```python
from build123d import *

# Parameters (mm, degrees)
BOSS_EXTRUDE1_DEPTH = 25
SHELL1_T            = -5
SKETCH3_W           = 5
SKETCH3_H           = 25
BOSS_EXTRUDE3_DEPTH = 5
CUT_EXTRUDE1_DEPTH  = 4.5


with BuildPart() as part:
    # Sketch1 → Boss-Extrude1 (new body)
    with BuildSketch(Plane(origin=(0, 0, 0), x_dir=(1, 0, 0), z_dir=(0, 1, 0))):
        Polygon((0, 42.5), (-36.806079661, 21.25), (-36.806079661, -21.25), (0, -42.5), (36.806079661, -21.25), (36.806079661, 21.25), align=None)
    extrude(amount=BOSS_EXTRUDE1_DEPTH)

    # Shell1
    shell1_openings = [part.faces().sort_by_distance(p)[0] for p in [
        (0, 25, 0),
        (-36.806079661, 12.5, 0),
    ]]
    offset(amount=SHELL1_T, openings=shell1_openings, kind=Kind.INTERSECTION)

    # Sketch3 → Boss-Extrude3 (add)
    with BuildSketch(Plane.XY.offset(-42.5)):
        with Locations((0, 12.5)):
            Rectangle(SKETCH3_W, SKETCH3_H)
    boss_extrude3 = extrude(amount=BOSS_EXTRUDE3_DEPTH)

    # Sketch4 → Cut-Extrude1 (cut)
    with BuildSketch(Plane(origin=(0, 0, -42.5), x_dir=(-1, 0, 0), z_dir=(0, 0, -1))):
        with BuildLine():
            ThreePointArc((0.573600046, 19.506352456), (1.318666007, 20.093843301), (1.6, 21))
            ThreePointArc((1.6, 21), (-0.906156699, 22.318666007), (-0.573600046, 19.506352456))
            ThreePointArc((-0.573600046, 19.506352456), (0, 19.71460041), (0.573600046, 19.506352456))
        make_face()
        with BuildLine():
            ThreePointArc((0.329089607, 2.434209455), (1.242284865, 2.991670533), (1.6, 4))
            ThreePointArc((1.6, 4), (-0.906156699, 5.318666007), (-0.573600046, 2.506352456))
            ThreePointArc((-0.573600046, 2.506352456), (-0.107313915, 2.657234104), (0.329089607, 2.434209455))
        make_face()
    cut_extrude1 = extrude(amount=-CUT_EXTRUDE1_DEPTH, mode=Mode.SUBTRACT)

    # Mirror1: Boss-Extrude3, Cut-Extrude1 across plane
    add(boss_extrude3.mirror(Plane.XY))
    add(cut_extrude1.mirror(Plane.XY), mode=Mode.SUBTRACT)


solid = part.part
```
Could you check a few things on this model? Use its own coordinates, in mm. A direction names the side the tool comes from. Give positions to 0.01 mm unless a question says otherwise; leave off trailing zeros. Write each loop counter-clockwise with the first axis right and the second up, starting at its lowest first coordinate (ties: lowest second). Pieces come first, ordered by that corner, then holes. Notation, with made-up numbers: (12.5, 65) - (34.5, 65) arc R18 cw to (34.5, 83) - close; hole circle Ø1 at (54.5, 80). An arc over 180 degrees is marked (long way). One line per item, written item: value. Start each with the question number.
Item 1: I'm going to push flat-ended pins straight in: pin 1 (0.7 mm diameter, centred on y = 7.5, z = -41.5, fed in from +X); pin 2 (0.9 mm diameter, centred on x = -0.5, y = 20.5, fed in from -Z); pin 3 (3.5 mm diameter, centred on x = 0, y = 21, fed in from -Z); pin 4 (1.5 mm diameter, centred on y = 3, z = 27, fed in from +X). Where does each tip first touch, or does it pass through?
Item 2: Imagine slicing it at D-D, the plane z = -33. List the corners of the cut face in (x, y) for me, and give its area (3 significant figures).
Item 3: Please list where these lines run through material, in increasing order: line 1 (Y direction, x = 0, z = -39); line 2 (X direction, y = 21, z = -41.45); line 3 (X direction, y = 16, z = -7.5). Write a range as from..to.
Item 4: Which directions (+Z, -Z, +X, -X, +Y, -Y) give clear straight access to the entire face, cutting with the end or side of a thin tool? Please do faces 4 (the face through (0, 21, 38)), 5 (the face through (-3, 5, -1)), 6 (the face through (0, 4, -38)).
Item 5: If we mould it in two halves opening along Y, with no side actions, what happens to faces 1 (the face through (22, 25, -25)), 2 (the face through (0, 4, 38)), 3 (the face through (-18.145, 14.86, -26.25))? For each: +Y half, -Y half, draft (parallel to the pull), parting line (faces both ways), or undercut.
Item 6: Imagine slicing it at A-A, the plane y = 10.5. List the corners of the cut face in (x, z) for me, and give its area (3 significant figures).
Item 7: Imagine slicing it at C-C, the plane z = 8. List the corners of the cut face in (x, y) for me.
Item 8: Imagine slicing it at B-B, the plane x = 27.5. List the corners of the cut face in (y, z) for me, and give its area (3 significant figures).
Geometry says:
1. pin 1: x = 2.5
1. pin 2: z = -38
1. pin 3: z = -42.5
1. pin 4: x = 28.15
2. outline: (-16.45, 0) - (16.45, 0) - (16.45, 25) - (6.45, 25) - (6.45, 5) - (-6.45, 5) - (-6.45, 25) - (-16.45, 25) - close
2. area: 565 mm^2
3. line 1: 0..2.64, 5.6..19.71, 22.6..25
3. line 2: -2.5..-1.6, 1.6..2.5
3. line 3: 31.81..36.81
4. face 4: +Z
4. face 5: +Y
4. face 6: -Z
5. face 1: +Y half
5. face 2: undercut
5. face 3: draft
6. outline: (-36.81, -21.25) - (-2.5, -41.06) - (-2.5, -42.5) - (2.5, -42.5) - (2.5, -41.06) - (36.81, -21.25) - (36.81, 21.25) - (2.5, 41.06) - (2.5, 42.5) - (-2.5, 42.5) - (-2.5, 41.06) - (-36.81, 21.25) - (-36.81, 15.48) - (0, 36.73) - (31.81, 18.36) - (31.81, -18.36) - (0, -36.73) - (-36.81, -15.48) - close
6. area: 1,030 mm^2
7. outline: (-36.81, 0) - (36.81, 0) - (36.81, 25) - (31.81, 25) - (31.81, 5) - (-36.81, 5) - close
8. outline: (0, -26.62) - (25, -26.62) - (25, -20.85) - (5, -20.85) - (5, 20.85) - (25, 20.85) - (25, 26.62) - (0, 26.62) - close
8. area: 497 mm^2
